```python
from build123d import *

# Parameters (mm, degrees)
BOSS_EXTRUDE1_DEPTH     = 7
SKETCH2_W               = 8
SKETCH2_H               = 4
BOSS_EXTRUDE2_DEPTH     = 16
FILLET1_RADIUS          = 4
FILLET1_LENGTH          = 4
SKETCH3_R               = 2
CUT_EXTRUDE1_DEPTH      = 16
SKETCH5_W               = 20
SKETCH5_H               = 7
SKETCH5_W_2             = 14
SKETCH5_W_3             = 6
CUT_EXTRUDE2_DEPTH      = 33
CUT_EXTRUDE3_DEPTH      = 73.387844283
CUT_EXTRUDE3_DEPTH_BACK = 73.387844283
SKETCH6_R               = 3
FILLET2_R               = 2


with BuildPart() as part:
    # Sketch1 → Boss-Extrude1 (new, symmetric)
    with BuildSketch(Plane.XY):
        with BuildLine():
            Line((0, 0), (0, 12))
            Line((0, 12), (-64, 12))
            ThreePointArc((-64, 12), (-70, 6), (-64, 0))
            Line((-64, 0), (0, 0))
        make_face()
    extrude(amount=BOSS_EXTRUDE1_DEPTH, both=True)

    # Sketch2 → Boss-Extrude2 (add)
    with BuildSketch(Plane(origin=(0, 0, 0), x_dir=(0, 0, -1), z_dir=(1, 0, 0))):
        with Locations((0, 6)):
            Rectangle(SKETCH2_W, SKETCH2_H)
    extrude(amount=BOSS_EXTRUDE2_DEPTH)

    # Fillet1: full round fillet: the end face becomes a half cylinder, R = half its width
    fillet1_face = Plane((16, 6, 0), x_dir=(0, -1, 0), z_dir=(1, 0, 0))  # on the end face: x along it, z out of the body
    fillet1_slab = fillet1_face.offset(-FILLET1_RADIUS / 2) * Box(FILLET1_LENGTH, 2 * FILLET1_RADIUS, FILLET1_RADIUS, mode=Mode.PRIVATE)  # the body's end, R deep
    fillet1_round = Plane((12, 6, 0), x_dir=(1, 0, 0), z_dir=(0, -1, 0)) * Cylinder(FILLET1_RADIUS, FILLET1_LENGTH, mode=Mode.PRIVATE)  # its axis R under the face
    add(fillet1_slab - fillet1_round, mode=Mode.SUBTRACT)

    # Sketch3 → Cut-Extrude1 (cut)
    with BuildSketch(Plane(origin=(0, 8, 0), x_dir=(1, 0, 0), z_dir=(0, 1, 0))):
        with Locations(Location((12, 0, 0), (0, 0, 270))):
            Circle(SKETCH3_R)
    extrude(amount=-CUT_EXTRUDE1_DEPTH, mode=Mode.SUBTRACT)

    # Sketch5 → Cut-Extrude2 (cut)
    with BuildSketch(Plane(origin=(0, 12, 0), x_dir=(1, 0, 0), z_dir=(0, 1, 0))):
        with Locations((-80, 0)):
            Rectangle(SKETCH5_W, SKETCH5_H)
        with Locations((-57, 0)):
            Rectangle(SKETCH5_W_2, SKETCH5_H)
        with Locations((-67, 0)):
            Rectangle(SKETCH5_W_3, SKETCH5_H)
    extrude(amount=-CUT_EXTRUDE2_DEPTH, mode=Mode.SUBTRACT)

    # Sketch6 → Cut-Extrude3 (cut, two sides: drawn at the far end of the back side and taken through both)
    with BuildSketch(Plane.XY.offset(7).offset(-CUT_EXTRUDE3_DEPTH_BACK)):
        with Locations((-64, 6)):
            Circle(SKETCH6_R)
    extrude(amount=CUT_EXTRUDE3_DEPTH + CUT_EXTRUDE3_DEPTH_BACK, mode=Mode.SUBTRACT)

    # Fillet2
    fillet2_edges = [part.edges().sort_by_distance(p)[0] for p in [
        (0, 4, 0),
        (0, 6, -4),
        (0, 8, 0),
        (0, 6, 4),
    ]]
    fillet(fillet2_edges, radius=FILLET2_R)


solid = part.part
```
Geometry: final body of the model. Coordinates: model frame, mm. A direction names the side the tool comes from. Round coordinates to 2 decimals unless told otherwise and drop trailing zeros. Loops run counter-clockwise (first coordinate to the right, second up) from the corner with the lowest first, then second, coordinate; pieces in that order, holes last. Notation, with made-up numbers: (2.25, 24.25) -> (56.25, 24.25) arc R25 cw to (56.25, 52.25) -> close; hole circle Ø2 at (-24.5, 53). An arc over 180 degrees is marked (long way). Use one line per item in the form item = value. Start each with the question number.
1) Section B-B on y = 11.25. Output: boundary loops of the cut face in (x, z).
2) First-contact query: P1, Ø4.5, axis at x = 8.5, y = 7, coming from the +Z side; P2, Ø3, axis at x = -39, z = 3.5, coming from the -Y side; P3, Ø4, axis at y = 1.5, z = 0.5, coming from the +X side; P4, Ø2, axis at y = 4, z = -1, coming from the -X side. Flat tips, straight axial feed; report the tip coordinate or a pass-through.
3) Access query for faces 1 (the flat face through (7, 6, 4)), 2 (the flat face through (7, 4, 0)), 3 (the flat face through (7, 6, -4)). Directions: +Z, -Z, +X, -X, +Y, -Y. A direction counts if a zero-diameter tool reaches every point of the face in a straight line with its end or side. Return the directions, or none.
4) Draft query along Z for faces 4 (the cylindrical face through (-66.4, 4.2, -5.3)), 5 (the flat face through (-58, 6, 3.5)), 6 (the cylindrical face through (14, 6, 0)), 7 (the cylindrical face through (0.35, 6.06, 4.87)). Return one class per face: released by +Z, released by -Z, zero draft, split by the parting line, or undercut.
5) Section A-A on z = 0. Output: boundary loops of the cut face in (x, y).
6) Line query: L1, parallel to Y at x = -64, z = -5.1; L2, parallel to Z at x = -54.5, y = 5; L3, parallel to X at y = 6.15, z = 0. Output: solid intervals per line, ascending.
Response:
q1.outline = (-66.9, -7) -> (0, -7) -> (0, 7) -> (-66.9, 7) -> (-66.9, 3.5) -> (-50, 3.5) -> (-50, -3.5) -> (-66.9, -3.5) -> close
q2.P1 = 4
q2.P2 = 0
q2.P3 = 0.68
q2.P4 = -50
q3.face_1 = +Z, +X, +Y, -Y
q3.face_2 = +Z, -Z, +X, -Y
q3.face_3 = -Z, +X, +Y, -Y
q4.face_4 = zero draft
q4.face_5 = undercut
q4.face_6 = undercut
q4.face_7 = released by +Z
q5.outline = (-50, 0) -> (0, 0) -> (0, 2) arc R2 cw to (2, 4) -> (10, 4) -> (10, 8) -> (2, 8) arc R2 cw to (0, 10) -> (0, 12) -> (-50, 12) -> close; (14, 4) -> (16, 4) -> (16, 8) -> (14, 8) -> close
q6.L1 = 0 to 3, 9 to 12
q6.L2 = -7 to -3.5, 3.5 to 7
q6.L3 = -50 to 10, 14 to 16
